Geometry check sheet. Reference: drawing and pictorial views, mm from the part's lowest x, y, z. Give positions to 0.01 mm unless a question says otherwise; leave off trailing zeros. Order: outer loops, then holes, each group sorted by start corner. A loop starts at its lowest first (then second) coordinate and runs counter-clockwise, first axis right, second up. Notation, with made-up numbers: M 66,-36 L 84,-36 A25 cw 84,-17 Z; hole C 87.5,-40 d8. An arc over 180 degrees is marked long. Answer as CSV lines item,"result". Start each with the question number.
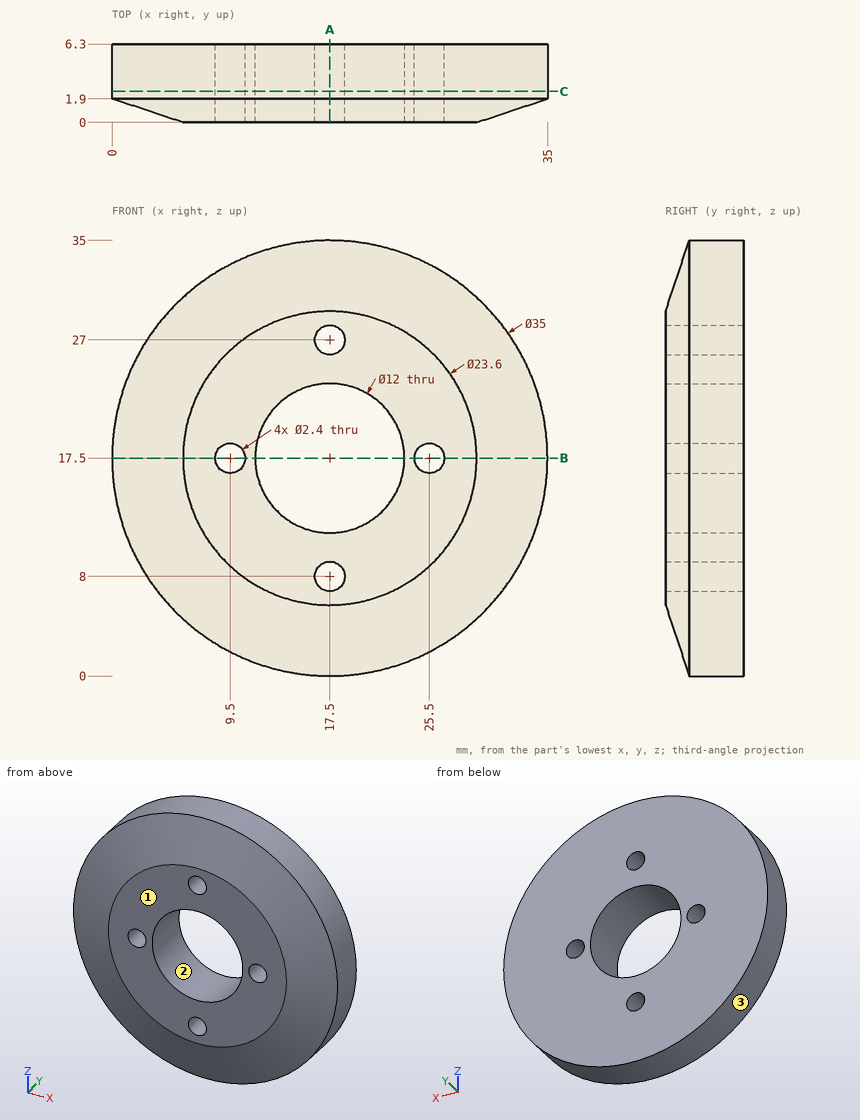
Item 1: Draft check along X on the marked faces 1, 2 and 3. Enter one of: pulls with the +X half, pulls with the -X half, needs draft (parallel to the pull), parting line crosses it, or undercut.
Item 2: Depth check by flat-ended pin: pin 1 Ø2 at (y, z) = (2.5, 3.5) entering from -X; pin 2 Ø1.5 at (y, z) = (2.5, 5) entering from -X. Enter the tip coordinate at first touch or a pass-through.
Item 3: Section check A-A on x = 17.5. Record the boundary of the cut face in (y, z), then the cut area to 3 significant figures.
Item 4: Section check B-B on z = 17.5. Record the boundary of the cut face in (x, y), then the cut area to 3 significant figures.
Item 5: Section check C-C on y = 2.5. Record the boundary of the cut face in (x, z).
Item 6: Scan lines: line 1 along Z through (x, y) = (17.5, 4.75); line 2 along X through (y, z) = (4.25, 17); line 3 along Z through (x, y) = (10, 3.25). Record each from-to range of solid material in increasing order.
Numbers:
1,face 1,"needs draft"
1,face 2,"undercut"
1,face 3,"parting line crosses it"
2,pin 1,"x = 5.78"
2,pin 2,"x = 4.53"
3,outline,"M 0,5.7 L 1.9,0 L 6.3,0 L 6.3,6.8 L 0,6.8 Z; M 0,9.2 L 6.3,9.2 L 6.3,11.5 L 0,11.5 Z; M 0,23.5 L 6.3,23.5 L 6.3,25.8 L 0,25.8 Z; M 0,28.2 L 6.3,28.2 L 6.3,35 L 1.9,35 L 0,29.3 Z"
3,area,"104 mm2"
4,outline,"M 0,1.9 L 5.7,0 L 8.3,0 L 8.3,6.3 L 0,6.3 Z; M 10.7,0 L 11.5,0 L 11.5,6.3 L 10.7,6.3 Z; M 23.5,0 L 24.3,0 L 24.3,6.3 L 23.5,6.3 Z; M 26.7,0 L 29.3,0 L 35,1.9 L 35,6.3 L 26.7,6.3 Z"
4,area,"104 mm2"
5,outline,"C 17.5,17.5 d35; hole C 9.5,17.5 d2.4; hole C 17.5,17.5 d12; hole C 17.5,8 d2.4; hole C 17.5,27 d2.4; hole C 25.5,17.5 d2.4"
6,line 1,"0 to 6.8, 9.2 to 11.5, 23.5 to 25.8, 28.2 to 35"
6,line 2,"0.01 to 8.41, 10.59 to 11.52, 23.48 to 24.41, 26.59 to 34.99"
6,line 3,"1.69 to 16.41, 18.59 to 33.31"
